from build123d import *

# Parameters (mm, degrees)
BOSS_EXTRUDE1_DEPTH        = 6.35
F_10_CLEARANCE_HOLE1_D     = 5.1054
F_10_CLEARANCE_HOLE1_DEPTH = 6.35
SKETCH5_R                  = 22.86
CUT_EXTRUDE1_DEPTH         = 7.35
CHAMFER1_SIZE              = 2.54
SKETCH6_W                  = 19.05
SKETCH6_H                  = 19.05
CUT_EXTRUDE2_DEPTH         = 6.35
FILLET1_R                  = 2.54
BOSS_EXTRUDE2_DEPTH        = 6.35
SKETCH8_W                  = 35.278450162
SKETCH8_H                  = 3.175
CUT_EXTRUDE3_DEPTH         = 2.032
CUT_EXTRUDE4_DEPTH         = 7.35
F_8_32_TAPPED_HOLE1_D      = 3.4544
F_8_32_TAPPED_HOLE1_DEPTH  = 6.35


with BuildPart() as part:
    # Sketch1 → Boss-Extrude1 (new body)
    with BuildSketch(Plane(origin=(0, 0, 0), x_dir=(1, 0, 0), z_dir=(0, 1, 0))):
        with BuildLine():
            Line((0, 0), (83.361013597, 0))
            ThreePointArc((83.361013597, 0), (87.71707766, -0.3763171), (91.944066022, -1.494117647))
            ThreePointArc((91.944066022, -1.494117647), (101.6, -3.175), (111.255933978, -1.494117647))
            ThreePointArc((111.255933978, -1.494117647), (115.48292234, -0.3763171), (119.838986403, 0))
            Line((119.838986403, 0), (203.2, 0))
            Line((203.2, 0), (203.2, 50.8))
            Line((203.2, 50.8), (119.838986403, 50.8))
            ThreePointArc((119.838986403, 50.8), (115.48292234, 51.1763171), (111.255933978, 52.294117647))
            ThreePointArc((111.255933978, 52.294117647), (101.6, 53.975), (91.944066022, 52.294117647))
            ThreePointArc((91.944066022, 52.294117647), (87.71707766, 51.1763171), (83.361013597, 50.8))
            Line((83.361013597, 50.8), (0, 50.8))
            Line((0, 50.8), (0, 0))
        make_face()
    extrude(amount=BOSS_EXTRUDE1_DEPTH)

    # #10 Clearance Hole1
    with Locations(Plane(origin=(0, 6.35, 0), x_dir=(1, 0, 0), z_dir=(0, 1, 0))):
        with Locations((12.7, 41.275), (12.7, 9.525), (190.5, 9.525), (190.5, 41.275)):
            Hole(F_10_CLEARANCE_HOLE1_D / 2, depth=F_10_CLEARANCE_HOLE1_DEPTH)

    # Sketch5 → Cut-Extrude1 (cut, through all)
    with BuildSketch(Plane(origin=(0, 6.35, 0), x_dir=(1, 0, 0), z_dir=(0, 1, 0))):
        with Locations((101.6, 25.4)):
            Circle(SKETCH5_R)
    extrude(amount=-CUT_EXTRUDE1_DEPTH, mode=Mode.SUBTRACT)

    # Chamfer1
    chamfer1_edges = [part.edges().sort_by_distance(p)[0] for p in [
        (0, 3.175, -50.8),
        (203.2, 3.175, -50.8),
        (203.2, 3.175, 0),
        (0, 3.175, 0),
    ]]
    chamfer(chamfer1_edges, length=CHAMFER1_SIZE)

    # Sketch6 → Cut-Extrude2 (cut)
    with BuildSketch(Plane(origin=(0, 6.35, 0), x_dir=(1, 0, 0), z_dir=(0, 1, 0))):
        Polygon((27.212667469, 46.0375), (81.006722435, 46.0375), (54.109694952, 27.333602302), align=None)
        Polygon((25.4, 43.430804459), (25.4, 7.369195541), (51.329089802, 25.4), align=None)
        Polygon((27.212667469, 4.7625), (81.006722435, 4.7625), (54.109694952, 23.466397698), align=None)
        with Locations((12.7, 25.4)):
            Rectangle(SKETCH6_W, SKETCH6_H)
        with BuildLine():
            Line((56.890300102, 25.4), (82.819389904, 43.430804459))
            ThreePointArc((82.819389904, 43.430804459), (75.565, 25.4), (82.819389904, 7.369195541))
            Line((82.819389904, 7.369195541), (56.890300102, 25.4))
        make_face()
        Polygon((151.870910198, 25.4), (177.8, 43.430804459), (177.8, 7.369195541), align=None)
        with BuildLine():
            Line((146.309699898, 25.4), (120.380610096, 7.369195541))
            ThreePointArc((120.380610096, 7.369195541), (127.635, 25.4), (120.380610096, 43.430804459))
            Line((120.380610096, 43.430804459), (146.309699898, 25.4))
        make_face()
        Polygon((175.987332531, 4.7625), (149.090305048, 23.466397698), (122.193277565, 4.7625), align=None)
        Polygon((122.193277565, 46.0375), (149.090305048, 27.333602302), (175.987332531, 46.0375), align=None)
        with Locations((190.5, 25.4)):
            Rectangle(SKETCH6_W, SKETCH6_H)
    extrude(amount=-CUT_EXTRUDE2_DEPTH, mode=Mode.SUBTRACT)

    # Fillet1
    fillet1_edges = [part.edges().sort_by_distance(p)[0] for p in [
        (180.975, 3.175, -34.925),
        (200.025, 3.175, -34.925),
        (200.025, 3.175, -15.875),
        (180.975, 3.175, -15.875),
        (120.380610096, 3.175, -7.369195541),
        (120.380610096, 3.175, -43.430804459),
        (146.309699898, 3.175, -25.4),
        (51.329089802, 3.175, -25.4),
        (25.4, 3.175, -7.369195541),
        (25.4, 3.175, -43.430804459),
        (82.819389904, 3.175, -43.430804459),
        (82.819389904, 3.175, -7.369195541),
        (56.890300102, 3.175, -25.4),
        (54.109694952, 3.175, -23.466397698),
        (81.006722435, 3.175, -4.7625),
        (27.212667469, 3.175, -4.7625),
        (3.175, 3.175, -15.875),
        (3.175, 3.175, -34.925),
        (22.225, 3.175, -34.925),
        (22.225, 3.175, -15.875),
        (122.193277565, 3.175, -46.0375),
        (175.987332531, 3.175, -46.0375),
        (149.090305048, 3.175, -27.333602302),
        (177.8, 3.175, -7.369195541),
        (151.870910198, 3.175, -25.4),
        (177.8, 3.175, -43.430804459),
        (175.987332531, 3.175, -4.7625),
        (122.193277565, 3.175, -4.7625),
        (149.090305048, 3.175, -23.466397698),
        (81.006722435, 3.175, -46.0375),
        (54.109694952, 3.175, -27.333602302),
        (27.212667469, 3.175, -46.0375),
    ]]
    fillet(fillet1_edges, radius=FILLET1_R)

    # Sketch7 → Boss-Extrude2 (add)
    with BuildSketch(Plane(origin=(0, 0, 0), x_dir=(1, 0, 0), z_dir=(0, 1, 0))):
        with BuildLine():
            Line((82.871537172, 61.799122114), (87.251420854, 71.191812981))
            ThreePointArc((87.251420854, 71.191812981), (88.423021822, 72.52776784), (90.128948078, 73.025))
            Line((90.128948078, 73.025), (94.51975, 73.025))
            Line((94.51975, 73.025), (96.04375, 71.501))
            Line((96.04375, 71.501), (96.04375, 53.429604188))
            ThreePointArc((96.04375, 53.429604188), (93.972748348, 52.938258065), (91.944066022, 52.294117647))
            ThreePointArc((91.944066022, 52.294117647), (87.71707766, 51.1763171), (83.361013597, 50.8))
            Line((83.361013597, 50.8), (65.606373829, 50.8))
            ThreePointArc((65.606373829, 50.8), (75.841931368, 53.783392957), (82.871537172, 61.799122114))
        make_face()
        with BuildLine():
            Line((120.328462828, 61.799122114), (115.948579146, 71.191812981))
            ThreePointArc((115.948579146, 71.191812981), (114.776978178, 72.52776784), (113.071051922, 73.025))
            Line((113.071051922, 73.025), (108.68025, 73.025))
            Line((108.68025, 73.025), (107.15625, 71.501))
            Line((107.15625, 71.501), (107.15625, 53.429604188))
            ThreePointArc((107.15625, 53.429604188), (109.227251652, 52.938258065), (111.255933978, 52.294117647))
            ThreePointArc((111.255933978, 52.294117647), (115.48292234, 51.1763171), (119.838986403, 50.8))
            Line((119.838986403, 50.8), (137.593626171, 50.8))
            ThreePointArc((137.593626171, 50.8), (127.358068632, 53.783392957), (120.328462828, 61.799122114))
        make_face()
    extrude(amount=BOSS_EXTRUDE2_DEPTH)

    # Sketch8 → Cut-Extrude3 (cut)
    with BuildSketch(Plane(origin=(0, 6.35, 0), x_dir=(1, 0, 0), z_dir=(0, 1, 0))):
        with Locations((101.6, 65.7225)):
            Rectangle(SKETCH8_W, SKETCH8_H)
    extrude(amount=-CUT_EXTRUDE3_DEPTH, mode=Mode.SUBTRACT)

    # Sketch9 → Cut-Extrude4 (cut, through all)
    with BuildSketch(Plane(origin=(0, 6.35, 0), x_dir=(1, 0, 0), z_dir=(0, 1, 0))):
        with BuildLine():
            Line((96.04375, 73.025), (107.15625, 73.025))
            Line((107.15625, 73.025), (107.15625, 53.467))
            ThreePointArc((107.15625, 53.467), (106.561090979, 52.030159021), (105.12425, 51.435))
            Line((105.12425, 51.435), (98.07575, 51.435))
            ThreePointArc((98.07575, 51.435), (96.638909021, 52.030159021), (96.04375, 53.467))
            Line((96.04375, 53.467), (96.04375, 73.025))
        make_face()
    extrude(amount=-CUT_EXTRUDE4_DEPTH, mode=Mode.SUBTRACT)

    # #8-32 Tapped Hole1
    with Locations(Plane(origin=(0, 6.35, 0), x_dir=(1, 0, 0), z_dir=(0, 1, 0))):
        with Locations((88.9, 65.7225), (114.3, 65.7225)):
            Hole(F_8_32_TAPPED_HOLE1_D / 2, depth=F_8_32_TAPPED_HOLE1_DEPTH)


solid = part.part
Model file for the job. Use its own axes, mm. A direction names the side the tool comes from. Round coordinates to 2 decimals unless told otherwise and drop trailing zeros. Loops run counter-clockwise (first coordinate to the right, second up) from the corner with the lowest first, then second, coordinate; pieces in that order, holes last. Notation, with made-up numbers: (23.25, -28.75) - (71.25, -28.75) arc R21 ccw to (71.25, -23.75) - close; hole circle Ø8 at (80, -36). An arc over 180 degrees is marked (long way). Write each question's results on one line, items separated by ' | '.
(1) Saw through at B-B, the plane z = -25.4. Count the separate pieces of the cut face and the enclosed holes in it, then the cut area to 3 significant figures.
Answer below:
separate pieces: 8 | enclosed holes: 0 | area: 240 mm^2
(2) Saw through at D-D, the plane x = 186. List the corners of the cut face in (y, z) (3 decimals), then the cut area to 3 significant figures.
Answer below:
outline: (0, -50.8) - (6.35, -50.8) - (6.35, -34.925) - (0, -34.925) - close; (0, -15.875) - (6.35, -15.875) - (6.35, 0) - (0, 0) - close | area: 202 mm^2
(3) Pin check, flat tips, straight feed: pin 1 (3 mm diameter, centred on x = 11, y = 4.5, fed in from -Z); pin 2 (1.6 mm diameter, centred on x = 117, y = 5.5, fed in from +Z). Stop position of each tip, or through.
Answer below:
pin 1: stops at z = -50.8 | pin 2: stops at z = 0.26
(4) 3-axis set-ups, long thin cutter, end or side, ignore diameter. For faces 5 (the cylindrical face through (75.315, 3.131, -6.5)), 6 (the flat face through (0, 3, -26)): which of +Z, -Z, +X, -X, +Y, -Y reach the whole face in a straight line?
Answer below:
face 5: +Y, -Y | face 6: +Z, -Z, -X, +Y, -Y
(5) Wall check: L1, parallel to Z at x = 190.5, y = 5.25 (3 decimals); L2, parallel to Z at x = 88.9, y = 3.5; L3, parallel to Z at x = 55, y = 3. Give the ranges that are in metal, low to high.
Answer below:
L1: z = -50.8 to -43.828, -38.722 to -34.925, -15.875 to -12.078, -6.972 to 0 | L2: z = -72.78 to -67.45, -64 to -44.41, -6.39 to 0.61 | L3: z = -50.8 to -46.04, -28.05 to -22.75, -4.76 to 0
(6) Mould opens along X. For faces 1 (the flat face through (111, 6.35, -70)), 2 (the flat face through (149, 3, -4.762)), 3 (the flat face through (13, 3, -15.875)), 4 (the flat face through (85.03, 3.13, -66.43)) say: released by +X, released by -X, zero draft, split by the parting line, or undercut.
Answer below:
face 1: zero draft | face 2: undercut | face 3: undercut | face 4: released by -X
(7) Saw through at A-A, the plane x = 101.6. List the corners of the cut face in (y, z) (3 decimals).
Answer below:
outline: (0, -51.435) - (6.35, -51.435) - (6.35, -48.26) - (0, -48.26) - close; (0, -2.54) - (6.35, -2.54) - (6.35, 3.175) - (0, 3.175) - close
(8) Saw through at C-C, the plane x = 12.7. List the corners of the cut face in (y, z) (3 decimals), then the cut area to 3 significant figures.
Answer below:
outline: (0, -50.8) - (6.35, -50.8) - (6.35, -43.828) - (0, -43.828) - close; (0, -38.722) - (6.35, -38.722) - (6.35, -34.925) - (0, -34.925) - close; (0, -15.875) - (6.35, -15.875) - (6.35, -12.078) - (0, -12.078) - close; (0, -6.972) - (6.35, -6.972) - (6.35, 0) - (0, 0) - close | area: 137 mm^2
